Could you check a few things on this model? Use its own coordinates, in mm. Face numbers are marked on the shaded views. Round coordinates to 2 decimals unless told otherwise and drop trailing zeros. Loops run counter-clockwise (first coordinate to the right, second up) from the corner with the lowest first, then second, coordinate; pieces in that order, holes last. Notation, with made-up numbers: M 11,42.25 L 29,42.25 A34 ccw 29,81.25 Z; hole C 23.5,23 d1. An arc over 180 degrees is marked long. One line per item, written item: value. Start each with the question number.
Q1. Thinking about a two-plate mould opening in Y: for the marked faces 1 and 2, which applies, released by +Y, released by -Y, zero draft, split by the parting line, or undercut?
Q2. Imagine slicing it at D-D (x = 18). Please give me the cut outline in (y, z), then the cut area to 3 significant figures.
Q3. I'm going to push flat-ended pins straight in: pin 1 Ø4.5 at (x, y) = (15, 0) entering from +Z; pin 2 Ø8 at (x, z) = (4.5, 4) entering from +Y; pin 3 Ø1.5 at (y, z) = (3, 4) entering from +X; pin 4 Ø5 at (x, z) = (10, 9.5) entering from -Y. Where does each tip first touch, or does it pass through?
Q4. Imagine slicing it at C-C (x = 15). Please give me the cut outline in (y, z), then the cut area to 3 significant figures.
Q5. Please list where these lines run through material, in increasing order: line 1 along Y through (x, z) = (15, 1.7); line 2 along X through (y, z) = (0, 5.5); line 3 along Y through (x, z) = (18.5, -1.5) (3 decimals).
Q6. Imagine slicing it at B-B (z = 1.75). Please give me the cut outline in (x, y).
Q7. Imagine slicing it at A-A (y = 0). Please give me the cut outline in (x, z).
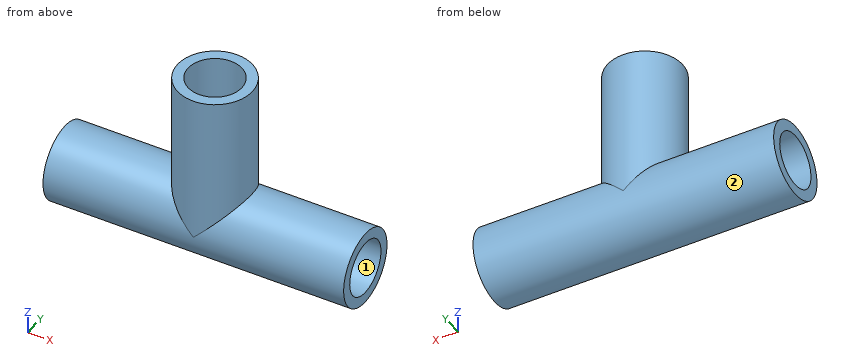
from build123d import *

# Parameters (mm, degrees)
SKETCH14_R          = 3.75
BOSS_EXTRUDE1_DEPTH = 30
SKETCH15_R          = 2.7
CUT_EXTRUDE4_DEPTH  = 30
SKETCH16_R          = 3.75
SKETCH16_R_2        = 2.7
BOSS_EXTRUDE2_DEPTH = 15
CUT_EXTRUDE5_START  = 25
SKETCH17_R          = 2.7
CUT_EXTRUDE5_DEPTH  = 25
SKETCH18_R          = 2.7
CUT_EXTRUDE6_DEPTH  = 25


with BuildPart() as part:
    # Sketch14 → Boss-Extrude1 (new body)
    with BuildSketch(Plane(origin=(0, 0, 0), x_dir=(0, 0, -1), z_dir=(1, 0, 0))):
        Circle(SKETCH14_R)
    extrude(amount=BOSS_EXTRUDE1_DEPTH)

    # Sketch15 → Cut-Extrude4 (cut)
    with BuildSketch(Plane(origin=(30, 0, 0), x_dir=(0, 0, -1), z_dir=(1, 0, 0))):
        Circle(SKETCH15_R)
    extrude(amount=-CUT_EXTRUDE4_DEPTH, mode=Mode.SUBTRACT)

    # Sketch16 → Boss-Extrude2 (add)
    with BuildSketch(Plane.XY):
        with Locations(Location((15, 0, 0), (0, 0, 90))):
            Circle(SKETCH16_R)
        with Locations((15, 0)):
            Circle(SKETCH16_R_2, mode=Mode.SUBTRACT)
    extrude(amount=BOSS_EXTRUDE2_DEPTH)

    # Sketch17 → Cut-Extrude5 (cut)
    with BuildSketch(Plane(origin=(0, 0, 0), x_dir=(0, 0, -1), z_dir=(1, 0, 0)).offset(CUT_EXTRUDE5_START)):
        Circle(SKETCH17_R)
    extrude(amount=-CUT_EXTRUDE5_DEPTH, mode=Mode.SUBTRACT)

    # Sketch18 → Cut-Extrude6 (cut)
    with BuildSketch(Plane.XY):
        with Locations(Location((15, 0, 0), (0, 0, 270))):
            Circle(SKETCH18_R)
    extrude(amount=CUT_EXTRUDE6_DEPTH, mode=Mode.SUBTRACT)


solid = part.part
Report:
1. face 1: undercut
1. face 2: split by the parting line
2. outline: M -2.25,3 A3.75 ccw long 2.25,3 L 2.25,15 L -2.25,15 Z; hole C 0,0 d5.4
2. area: 73.0 mm²
3. pin 1: stops at z = -1.49
3. pin 2: stops at y = 3.75
3. pin 3: stops at x = 18
3. pin 4: stops at y = -2.8
4. outline: M -3.75,0 A3.75 ccw 3.75,0 L 3.75,15 L 2.7,15 L 2.7,0 A2.7 cw -2.7,0 L -2.7,15 L -3.75,15 Z
4. area: 42.1 mm²
5. line 1: y = -3.75 to -2.7, 2.7 to 3.75
5. line 2: x = 11.25 to 12.3, 17.7 to 18.75
5. line 3: y = -3.437 to -2.245, 2.245 to 3.437
6. outline: M 0,-3.32 L 13.25,-3.32 A3.75 ccw 16.75,-3.32 L 30,-3.32 L 30,-2.06 L 16.75,-2.06 A2.7 cw 13.25,-2.06 L 0,-2.06 Z; M 0,2.06 L 13.25,2.06 A2.7 cw 16.75,2.06 L 30,2.06 L 30,3.32 L 16.75,3.32 A3.75 ccw 13.25,3.32 L 0,3.32 Z
7. outline: M 0,-3.75 L 30,-3.75 L 30,-2.7 L 0,-2.7 Z; M 0,2.7 L 12.3,2.7 L 12.3,15 L 11.25,15 L 11.25,3.75 L 0,3.75 Z; M 17.7,2.7 L 30,2.7 L 30,3.75 L 18.75,3.75 L 18.75,15 L 17.7,15 Z
